```python
from build123d import *

# Parameters (mm, degrees)
F0_R     = 10.3251
F1_DEPTH = 7.9375
F2_R     = 9.92251
F3_DEPTH = 7.9375
F4_R     = 6.35


# Not quite as in the source:
# - a pattern or mirror of a feature is missing from the dataset's text; its kind, count and spacing are read off the source's solid


with BuildPart() as f1:
    # F0 (on Top) → F1 (new body)
    with BuildSketch(Plane.XY):
        with BuildLine():
            Line((0, 73.025), (0, 0))
            Line((0, 0), (57.15, 0))
            Line((57.15, 0), (57.15, 14.2875))
            Line((57.15, 14.2875), (111.125, 14.2875))
            ThreePointArc((111.125, 14.2875), (133.35, 36.5125), (111.125, 58.7375))
            Line((111.125, 58.7375), (57.15, 58.7375))
            Line((57.15, 58.7375), (57.15, 73.025))
            Line((57.15, 73.025), (0, 73.025))
        make_face()
        with Locations((73.025, 36.5125)):
            Circle(F0_R, mode=Mode.SUBTRACT)
        with Locations((111.125, 36.5125)):
            Circle(F0_R, mode=Mode.SUBTRACT)
    extrude(amount=F1_DEPTH)

    # F2 (on Front) → F3 (join)
    with BuildSketch(Plane.XZ):
        with BuildLine():
            Line((0, 44.45), (0, 0))
            Line((0, 0), (57.15, 0))
            Line((57.15, 0), (57.15, 44.45))
            ThreePointArc((57.15, 44.45), (28.575, 73.025), (0, 44.45))
        make_face()
        with Locations((28.575, 44.45)):
            Circle(F2_R, mode=Mode.SUBTRACT)
    f3 = extrude(amount=-F3_DEPTH)

    # F3_copies: F3 across plane
    add(f3.mirror(Plane.ZX.offset(36.5125)))

    # F4
    f4_edges = [f1.edges().sort_by_distance(p)[0] for p in [
        (57.15, 14.2875, 3.96875),
        (57.15, 58.7375, 3.96875),
    ]]
    fillet(f4_edges, radius=F4_R)


solid = f1.part
```
Can you work these out from the model? Positions are in its coordinate system, mm. A direction names the side the tool comes from. Give positions to 0.01 mm unless a question says otherwise; leave off trailing zeros. Write each loop counter-clockwise with the first axis right and the second up, starting at its lowest first coordinate (ties: lowest second). Pieces come first, ordered by that corner, then holes. Notation, with made-up numbers: (20, -22) -> (64, -22) arc R12 ccw to (64, -3) -> close; hole circle Ø2 at (15.25, 80). An arc over 180 degrees is marked (long way). Write item = value, one per line.
(1) Suppose I cut it at D-D on y = 41. Write out the boundary of the cut face in (x, z).
Worked out:
outline = (0, 0) -> (63.73, 0) -> (63.73, 7.94) -> (0, 7.94) -> close; (82.32, 0) -> (101.83, 0) -> (101.83, 7.94) -> (82.32, 7.94) -> close; (120.42, 0) -> (132.89, 0) -> (132.89, 7.94) -> (120.42, 7.94) -> close
(2) For faces 1 (the face through (120.973, 39.614, 3.913)), 2 (the face through (26.424, 3.913, 34.763)), 3 (the face through (57.15, 69, 22)), 4 (the face through (87, 14.288, 4)), 5 (the face through (28, 65.088, 34)), which set-ups out of +Z, -Z, +X, -X, +Y, -Y let a thin tool reach every point of the face, with its end or its side?
Worked out:
face_1 = +Z, -Z
face_2 = +Y, -Y
face_3 = +Z, -Z, +X, +Y
face_4 = +Z, -Z, +X, -Y
face_5 = +Z, +X, -X
(3) Suppose I cut it at C-C on x = 105.5. Write out the boundary of the cut face in (y, z).
Worked out:
outline = (14.29, 0) -> (27.85, 0) -> (27.85, 7.94) -> (14.29, 7.94) -> close; (45.17, 0) -> (58.74, 0) -> (58.74, 7.94) -> (45.17, 7.94) -> close
(4) I need wall thicknesses on probe 1 along Y at (x, z) = (50, 62) (1 decimal); probe 2 along Z at (x, y) = (43.5, 26); probe 3 along X at (y, z) = (69, 4.5). Which ranges of each line are inside material? Lowest first, please. Write a range as from..to.
Worked out:
probe_1 = 0..7.9, 65.1..73
probe_2 = 0..7.94
probe_3 = 0..57.15
(5) I'm going to push flat-ended pins straight in: P1, Ø8.5, axis at y = 67.5, z = 22.5, coming from the +X side; P2, Ø2.5, axis at x = 83, z = 4.5, coming from the -Y side; P3, Ø2, axis at x = 37.5, y = 11.5, coming from the +Z side. Where does each tip first touch, or does it pass through?
Worked out:
P1 = 57.15
P2 = 14.29
P3 = 7.94
(6) Thinking about a two-plate mould opening in Y: for faces 6 (the face through (59.06, 12.477, 4.024)), 7 (the face through (51, 37, 7.938)), 8 (the face through (29.2, 69.11, 73.02)), which applies, released by +Y, released by -Y, zero draft, split by the parting line, or undercut?
Worked out:
face_6 = released by -Y
face_7 = undercut
face_8 = zero draft
(7) Suppose I cut it at B-B on z = 42. Count the separate pieces of the cut face and the enclosed holes in it, then the cut area to 3 significant figures.
Worked out:
separate_pieces = 4
enclosed_holes = 0
area = 602 mm^2
